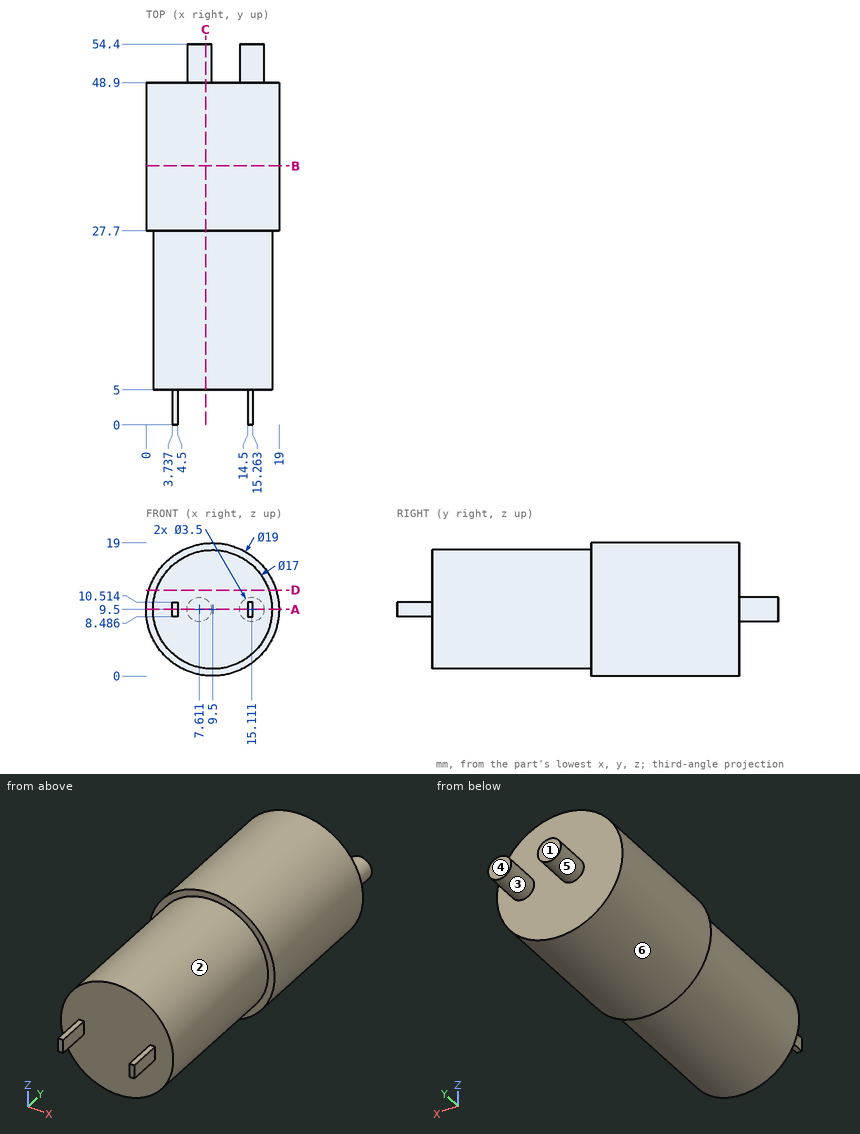
Geometry check sheet. Reference: drawing and pictorial views, mm from the part's lowest x, y, z. A direction names the side the tool comes from. Give positions to 0.01 mm unless a question says otherwise; leave off trailing zeros. Write each loop counter-clockwise with the first axis right and the second up, starting at its lowest first coordinate (ties: lowest second). Pieces come first, ordered by that corner, then holes. Notation, with made-up numbers: (75, -26) - (92, -26) arc R23 cw to (92, 4) - close; hole circle Ø7 at (-11, -11.5). An arc over 180 degrees is marked (long way). Put each result on its own line as item: value.
Q1. Section check C-C on x = 8.5. Record the cut outline in (y, z).
Result:
outline: (5, 1.06) - (27.7, 1.06) - (27.7, 0.05) - (48.9, 0.05) - (48.9, 7.99) - (54.4, 7.99) - (54.4, 11.01) - (48.9, 11.01) - (48.9, 18.95) - (27.7, 18.95) - (27.7, 17.94) - (5, 17.94) - close
Q2. Section check B-B on y = 37. Record the cut outline in (x, z).
Result:
outline: circle Ø19 at (9.5, 9.5)
Q3. Set-up check for the marked faces 1 and 2: record each of +Z, -Z, +X, -X, +Y, -Y from which the full face is reachable in a straight line by a thin tool's end or side.
Result:
face 1: +Z, -Z, +X, -X, +Y
face 2: -Y
Q4. Scan lines: probe 1 along Y at (x, z) = (12.25, 17.75); probe 2 along Y at (x, z) = (14.5, 14); probe 3 along Z at (x, y) = (12.75, 42.5). Record each from-to range of solid material in increasing order. Write a range as from..to.
Result:
probe 1: 27.7..48.9
probe 2: 5..48.9
probe 3: 0.57..18.43
Q5. Depth check by flat-ended pin: P1, Ø0.6, axis at x = 4, y = 3.5, coming from the +Z side; P2, Ø8, axis at y = 30, z = 4.5, coming from the -X side; P3, Ø1.6, axis at y = 1.5, z = 9.5, coming from the -X side. Enter the tip coordinate at first touch or a pass-through.
Result:
P1: z = 10.51
P2: x = 0.05
P3: x = 3.74
Q6. Section check A-A on z = 9.5. Record the cut outline in (x, y).
Result:
outline: (0, 27.7) - (1, 27.7) - (1, 5) - (3.74, 5) - (3.74, 0) - (4.5, 0) - (4.5, 5) - (14.5, 5) - (14.5, 0) - (15.26, 0) - (15.26, 5) - (18, 5) - (18, 27.7) - (19, 27.7) - (19, 48.9) - (16.86, 48.9) - (16.86, 54.4) - (13.36, 54.4) - (13.36, 48.9) - (9.36, 48.9) - (9.36, 54.4) - (5.86, 54.4) - (5.86, 48.9) - (0, 48.9) - close
Q7. Section check D-D on z = 12.25. Record the cut outline in (x, y).
Result:
outline: (0.41, 27.7) - (1.46, 27.7) - (1.46, 5) - (17.54, 5) - (17.54, 27.7) - (18.59, 27.7) - (18.59, 48.9) - (0.41, 48.9) - close
Q8. Mould release check, pull along X, two halves, no side actions. Record for the marked faces 3, 4, 5 and 6: released by +X, released by -X, zero draft, split by the parting line, or undercut.
Result:
face 3: undercut
face 4: zero draft
face 5: undercut
face 6: split by the parting line
